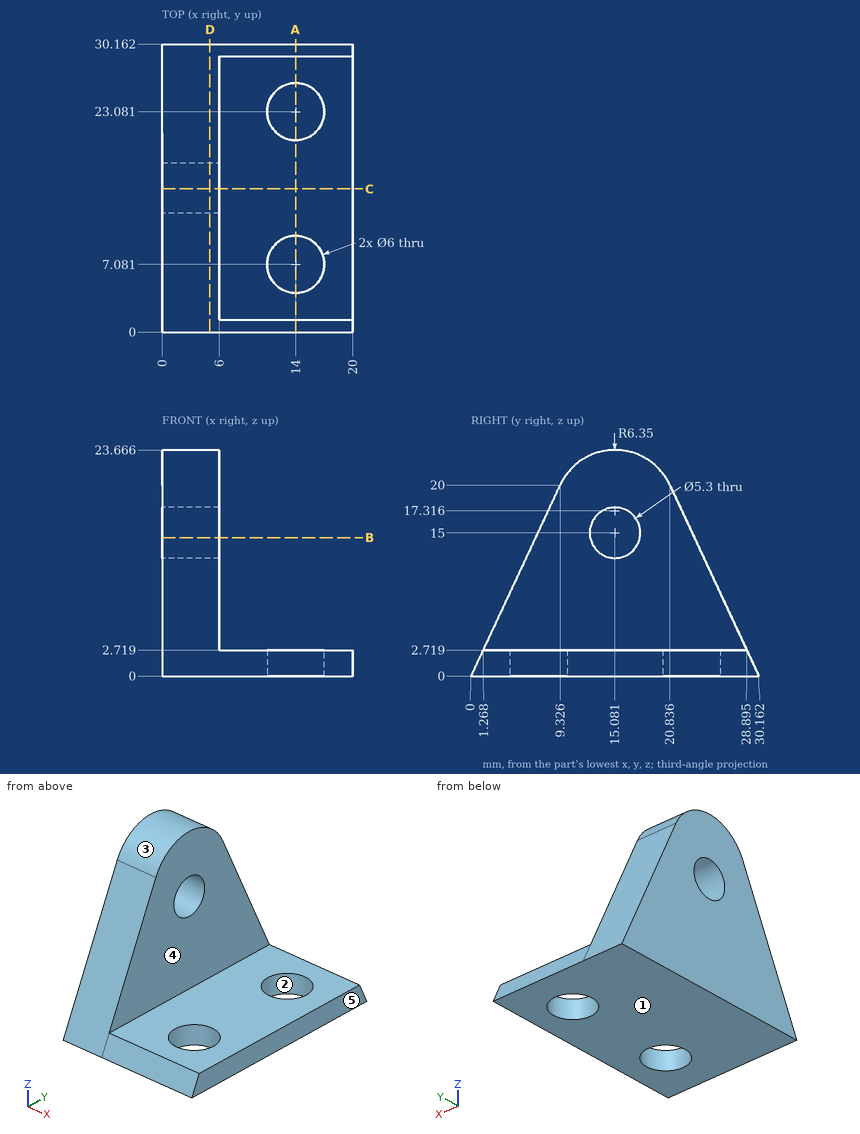
Input: dimensioned drawing with shaded views. Units: mm. Origin: part minimum x, y, z. A direction names the side the tool comes from. Coordinates: 2 decimals unless noted, no trailing zeros. Loops run counter-clockwise (first coordinate to the right, second up) from the corner with the lowest first, then second, coordinate; pieces in that order, holes last. Notation, with made-up numbers: M 38.25,34 L 52.25,34 A25 cw 52.25,59 Z; hole C 42.25,12.5 d8. An arc over 180 degrees is marked long. One line per item, written item: value.
(1) Section C-C (y = 15). Output: boundary loops of the cut face in (x, z) (1 decimal), and give its area (3 significant figures).
Filled in:
outline: M 0,0 L 20,0 L 20,2.7 L 6,2.7 L 6,12.4 L 0,12.4 Z; M 0,17.6 L 6,17.6 L 6,23.7 L 0,23.7 Z
area: 148 mm^2
(2) Section B-B (z = 14.5). Output: boundary loops of the cut face in (x, y), and give its area (3 significant figures).
Filled in:
outline: M 0,6.76 L 6,6.76 L 6,12.48 L 0,12.48 Z; M 0,17.68 L 6,17.68 L 6,23.4 L 0,23.4 Z
area: 68.6 mm^2
(3) Section D-D (x = 5). Output: boundary loops of the cut face in (y, z).
Filled in:
outline: M 0,0 L 30.16,0 L 20.84,20 A6.35 ccw 9.33,20 Z; hole C 15.08,15 d5.3
(4) Reachability of the marked faces 4 and 5 from +Z, -Z, +X, -X, +Y, -Y: full face, straight path, thin tool, end or side. Return the list, or none.
Filled in:
face 4: +Z, +X, +Y, -Y
face 5: +Z, -Z, +X, +Y, -Y
(5) Section A-A (x = 14). Output: boundary loops of the cut face in (y, z) (1 decimal).
Filled in:
outline: M 0,0 L 4.1,0 L 4.1,2.7 L 1.3,2.7 Z; M 10.1,0 L 20.1,0 L 20.1,2.7 L 10.1,2.7 Z; M 26.1,0 L 30.2,0 L 28.9,2.7 L 26.1,2.7 Z
(6) Pull-direction query (Y, two-part tool) for the marked faces 1, 2 and 3; classes: +Y half, -Y half, draft (parallel to the pull), parting line (faces both ways), or undercut.
Filled in:
face 1: draft
face 2: undercut
face 3: parting line
(7) Line query: line 1 along Y through (x, z) = (14, 0.75); line 2 along Y through (x, z) = (13.5, 2.25); line 3 along X through (y, z) = (19, 5.25). Output: solid intervals per line, ascending. Write a range as from..to.
Filled in:
line 1: 0.35..4.08, 10.08..20.08, 26.08..29.81
line 2: 1.05..4.12, 10.04..20.12, 26.04..29.11
line 3: 0..6
(8) Pin query (flat end, axial travel): pin 1 (2 mm diameter, centred on x = 9.5, y = 19, fed in from +Z); pin 2 (5 mm diameter, centred on y = 15.08, z = 15, fed in from -X); pin 3 (1 mm diameter, centred on x = 14.5, z = 2.5, fed in from -Y); pin 4 (6.5 mm diameter, centred on y = 15, z = 12.5, fed in from +X). Return the tip coordinate at first contact, or that it passes through.
Filled in:
pin 1: z = 2.72
pin 2: through
pin 3: y = 0.93
pin 4: x = 6
